Work out the finished part from the listing and answer in its coordinate system (mm). Face numbers are marked on the shaded views. A direction names the side the tool comes from. Give positions to 0.01 mm unless a question says otherwise; leave off trailing zeros. Write each loop counter-clockwise with the first axis right and the second up, starting at its lowest first coordinate (ties: lowest second). Pieces come first, ordered by that corner, then holes.
1) Find section C-C (y = 13.5). Determine the outline of the cut face in (x, z), plus the area to 3 significant figures.
2) Straight lines are drawn through the part: probe 1 along X at (y, z) = (1.65, 30); probe 2 along Z at (x, y) = (14, 44). For each, find the intervals that lie inside material, in ascending order.
3) Find section D-D (x = 19.5). Determine the outline of the cut face in (y, z).
4) A tool of negligible diameter and unlimited length cuts with its end or side. For the marked faces 1, 2 and 3, from which of +Z, -Z, +X, -X, +Y, -Y can it reach the whole face along a straight path? Write none if from no direction.
5) Given pin 1 Ø5.5 at (x, z) = (15.5, 3) entering from -Y; pin 2 Ø6 at (x, y) = (16, 8) entering from +Z; pin 3 Ø2 at (y, z) = (4.5, 13) entering from +X; pin 4 Ø1.5 at (x, y) = (17.5, 17.5) entering from -Z, each flat-ended and moving along its own axis, determine where each tip first touches the part or whether it passes through.
6) Find section B-B (x = 5). Determine the outline of the cut face in (y, z), plus the area to 3 significant figures.
7) Find section A-A (z = 10). Determine the outline of the cut face in (x, y), plus the area to 3 significant figures.
```python
from build123d import *

# Parameters (mm, degrees)
BOSS_EXTRUDE1_DEPTH = 5
SKETCH2_W           = 10
SKETCH2_H           = 5
BOSS_EXTRUDE2_DEPTH = 30
SKETCH3_R           = 1.5
CUT_EXTRUDE1_DEPTH  = 5
SKETCH4_W           = 20
SKETCH4_H           = 7
CUT_EXTRUDE2_DEPTH  = 5


with BuildPart() as part:
    # Sketch1 → Boss-Extrude1 (new body)
    with BuildSketch(Plane.XY):
        Polygon((0, 35), (8.660254038, 50), (21.339745962, 50), (30, 35), (30, 0), (0, 0), align=None)
    extrude(amount=BOSS_EXTRUDE1_DEPTH)

    # Sketch2 → Boss-Extrude2 (add)
    with BuildSketch(Plane.XY.offset(5)):
        with Locations((5, 2.5)):
            Rectangle(SKETCH2_W, SKETCH2_H)
    extrude(amount=BOSS_EXTRUDE2_DEPTH)

    # Sketch3 → Cut-Extrude1 (cut)
    with BuildSketch(Plane(origin=(0, 5, 0), x_dir=(1, 0, 0), z_dir=(0, 1, 0))):
        with Locations(Location((5, -10, 0), (0, 0, 270))):
            Circle(SKETCH3_R)
        with Locations(Location((5, -30, 0), (0, 0, 270))):
            Circle(SKETCH3_R)
    extrude(amount=-CUT_EXTRUDE1_DEPTH, mode=Mode.SUBTRACT)

    # Sketch4 → Cut-Extrude2 (cut)
    with BuildSketch(Plane.XY.offset(5)):
        with Locations((20, 3.5)):
            Rectangle(SKETCH4_W, SKETCH4_H)
    extrude(amount=-CUT_EXTRUDE2_DEPTH, mode=Mode.SUBTRACT)


solid = part.part
```
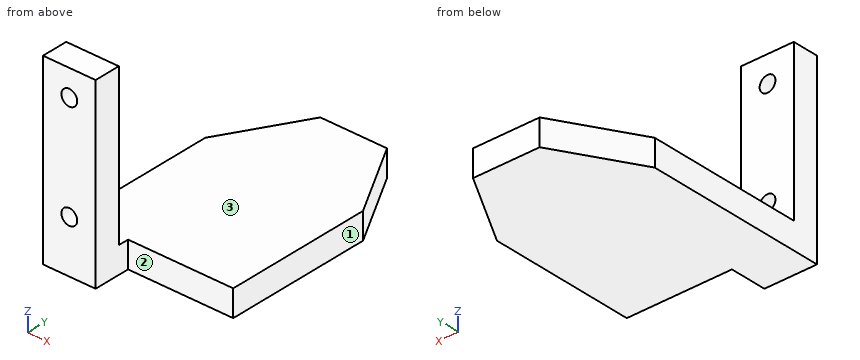
Results:
1. outline: (0, 0) - (30, 0) - (30, 5) - (0, 5) - close
1. area: 150 mm2
2. probe 1: x = 0 to 3.5, 6.5 to 10
2. probe 2: z = 0 to 5
3. outline: (7, 0) - (50, 0) - (50, 5) - (7, 5) - close
4. face 1: +Z, -Z, +X, +Y, -Y
4. face 2: +Z, -Z, +X, -Y
4. face 3: +Z, +X, -X, +Y
5. pin 1: stops at y = 7
5. pin 2: stops at z = 5
5. pin 3: stops at x = 10
5. pin 4: stops at z = 0
6. outline: (0, 0) - (43.66, 0) - (43.66, 5) - (5, 5) - (5, 8.5) - (0, 8.5) - close; (0, 11.5) - (5, 11.5) - (5, 28.5) - (0, 28.5) - close; (0, 31.5) - (5, 31.5) - (5, 35) - (0, 35) - close
6. area: 338 mm2
7. outline: (0, 0) - (3.5, 0) - (3.5, 5) - (0, 5) - close; (6.5, 0) - (10, 0) - (10, 5) - (6.5, 5) - close
7. area: 35.0 mm2
